Could you check a few things on this model? Use its own coordinates, in mm. Face numbers are marked on the shaded views. A direction names the side the tool comes from. Give positions to 0.01 mm unless a question says otherwise; leave off trailing zeros. Order: outer loops, then holes, each group sorted by start corner. A loop starts at its lowest first (then second) coordinate and runs counter-clockwise, first axis right, second up. Notation, with made-up numbers: M 48,27 L 58,27 A12 ccw 58,42 Z; hole C -11,37 d9. An arc over 180 degrees is marked long. Use a Markdown table: item, result. Add a question column.
Item 1: Suppose I cut it at A-A on z = 75. Write out the boundary of the cut face in (x, y).
Item 2: Suppose I cut it at B-B on z = 13. Write out the boundary of the cut face in (x, y), plus the area to 3 significant figures.
Item 3: For the marked faces 1 and 2, which set-ups out of +Z, -Z, +X, -X, +Y, -Y let a thin tool reach every point of the face, with its end or its side?
Item 4: If I drill on L1, parallel to X at y = -0.75, z = 12.5; L2, parallel to Z at x = 1.5, y = 4.25; L3, parallel to X at y = 1.25, z = 15, over which ranges is the centre line in solid material (lowest first)? Write a range as from..to.
Item 5: I'm going to push flat-ended pins straight in: pin 1 Ø1.5 at (y, z) = (1, 73) entering from +X; pin 2 Ø2 at (y, z) = (1.5, 13) entering from +X; pin 3 Ø1.5 at (x, z) = (-0.5, 41) entering from -Y. Where does each tip first touch, or does it pass through?
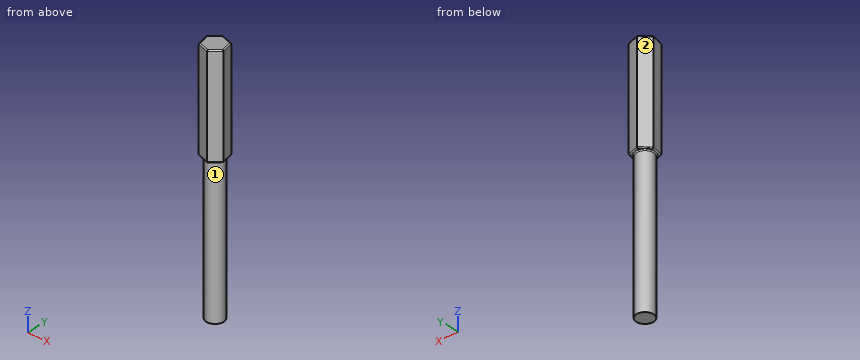
from build123d import *

# Parameters (mm, degrees)
BOSS_EXTRUDE1_DEPTH      = 85
BOSS_EXTRUDE1_DEPTH_BACK = 30
SKETCH1_R                = 4
BOSS_EXTRUDE2_DEPTH      = 47
FILLET1_R                = 0.5


with BuildPart() as part:
    # Sketch1 → Boss-Extrude1 (new, two sides: drawn at the far end of the back side and taken through both)
    with BuildSketch(Plane.XY.offset(-BOSS_EXTRUDE1_DEPTH_BACK)):
        Circle(SKETCH1_R)
    extrude(amount=BOSS_EXTRUDE1_DEPTH + BOSS_EXTRUDE1_DEPTH_BACK)

    # Sketch2 → Boss-Extrude2 (add)
    with BuildSketch(Plane.XY.offset(85)):
        Polygon((5.513335358, -1.713612138), (4.240699323, 3.917882411), (-1.272636036, 5.631494549), (-5.513335358, 1.713612138), (-4.240699323, -3.917882411), (1.272636036, -5.631494549), align=None)
    extrude(amount=-BOSS_EXTRUDE2_DEPTH)

    # Fillet1
    fillet1_edges = [part.edges().sort_by_distance(p)[0] for p in [
        (1.484031644, 4.77468848, 38),
        (4.877017341, 1.102135137, 38),
        (3.392985697, -3.672553343, 85),
        (4.877017341, 1.102135137, 85),
        (1.484031644, 4.77468848, 85),
        (-3.392985697, 3.672553343, 85),
        (-4.877017341, -1.102135137, 85),
        (-1.484031644, -4.77468848, 85),
        (-4, 0, 38),
        (3.392985697, -3.672553343, 38),
        (-1.484031644, -4.77468848, 38),
        (-4.877017341, -1.102135137, 38),
        (-3.392985697, 3.672553343, 38),
    ]]
    fillet(fillet1_edges, radius=FILLET1_R - 0.0001)  # a hair under: the kernel refuses the full size


solid = part.part
Findings below:
| question | item | result |
|---|---|---|
| 1 | outline | M -5.51,1.71 L -4.24,-3.92 L 1.27,-5.63 L 5.51,-1.71 L 4.24,3.92 L -1.27,5.63 Z |
| 2 | outline | C 0,0 d8 |
| 2 | area | 50.3 mm^2 |
| 3 | face 1 | -Z |
| 3 | face 2 | +Z, -Z, -X, +Y |
| 4 | L1 | x = -3.93..3.93 |
| 4 | L2 | z = 38..85 |
| 4 | L3 | x = -3.8..3.8 |
| 5 | pin 1 | stops at x = 5.07 |
| 5 | pin 2 | stops at x = 3.97 |
| 5 | pin 3 | stops at y = -5.31 |
